Here's how the part is built. I have some questions about the finished solid (model axes, mm). Face numbers are marked on the shaded views. A direction names the side the tool comes from. Round coordinates to 2 decimals unless told otherwise and drop trailing zeros. Order: outer loops, then holes, each group sorted by start corner. A loop starts at its lowest first (then second) coordinate and runs counter-clockwise, first axis right, second up. Notation, with made-up numbers: (47, 11) - (105, 11) arc R26 ccw to (105, 42) - close; hole circle Ø10 at (42, 5.5). An arc over 180 degrees is marked (long way). One line per item, written item: value.
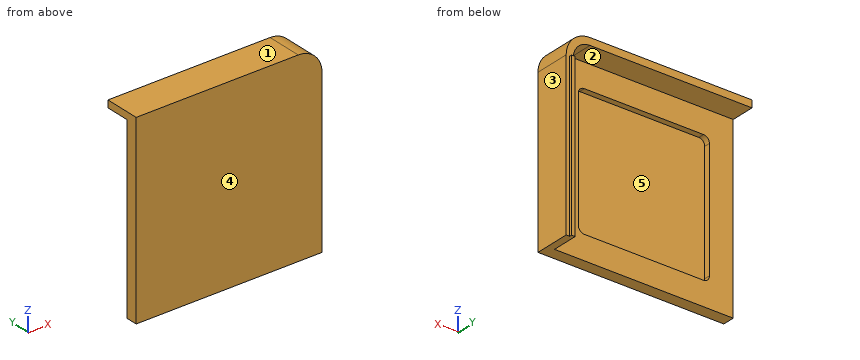
from build123d import *

# Parameters (mm, degrees)
SKIZZE9_W               = 156
SKIZZE9_H               = 156
SKIZZE9_W_2             = 110
SKIZZE9_H_2             = 110
LINEAR_AUSTRAGEN4_DEPTH = 5
VERRUNDUNG5_R           = 5
SKIZZE10_W              = 156
SKIZZE10_H              = 156
LINEAR_AUSTRAGEN5_DEPTH = 5
LINEAR_AUSTRAGEN6_DEPTH = 20
VERRUNDUNG6_R           = 20
VERRUNDUNG7_R           = 14
SKIZZE12_W              = 3
SKIZZE12_H              = 136
LINEAR_AUSTRAGEN7_DEPTH = 2


with BuildPart() as part:
    # Skizze9 → Linear austragen4 (new body)
    with BuildSketch(Plane(origin=(0, 0, 0), x_dir=(1, 0, 0), z_dir=(0, 1, 0))):
        with Locations((78, 78)):
            Rectangle(SKIZZE9_W, SKIZZE9_H)
        with Locations((75, 81)):
            Rectangle(SKIZZE9_W_2, SKIZZE9_H_2, mode=Mode.SUBTRACT)
    extrude(amount=LINEAR_AUSTRAGEN4_DEPTH)

    # Verrundung5
    verrundung5_edges = [part.edges().sort_by_distance(p)[0] for p in [
        (20, 2.5, -136),
        (20, 2.5, -26),
        (130, 2.5, -26),
        (130, 2.5, -136),
    ]]
    fillet(verrundung5_edges, radius=VERRUNDUNG5_R)

    # Skizze10 → Linear austragen5 (add)
    with BuildSketch(Plane.XZ):
        with Locations((78, -78)):
            Rectangle(SKIZZE10_W, SKIZZE10_H)
    extrude(amount=LINEAR_AUSTRAGEN5_DEPTH)

    # Skizze11 → Linear austragen6 (add)
    with BuildSketch(Plane(origin=(0, 5, 0), x_dir=(1, 0, 0), z_dir=(0, 1, 0))):
        Polygon((0, 0), (156, 0), (156, 156), (150, 156), (150, 6), (0, 6), align=None)
    extrude(amount=LINEAR_AUSTRAGEN6_DEPTH)

    # Verrundung6
    verrundung6_edges = [part.edges().sort_by_distance(p)[0] for p in [
        (156, 10, 0),
    ]]
    fillet(verrundung6_edges, radius=VERRUNDUNG6_R)

    # Verrundung7
    verrundung7_edges = [part.edges().sort_by_distance(p)[0] for p in [
        (150, 15, -6),
    ]]
    fillet(verrundung7_edges, radius=VERRUNDUNG7_R)

    # Skizze12 → Linear austragen7 (add)
    with BuildSketch(Plane(origin=(0, 25, 0), x_dir=(1, 0, 0), z_dir=(0, 1, 0))):
        with Locations((151.5, 88)):
            Rectangle(SKIZZE12_W, SKIZZE12_H)
    extrude(amount=LINEAR_AUSTRAGEN7_DEPTH)


solid = part.part
Q1. If we section it at A-A, the plane z = -111: Please give me the cut outline in (x, y).
Results list:
outline: (0, -5) - (156, -5) - (156, 25) - (153, 25) - (153, 27) - (150, 27) - (150, 5) - (130, 5) - (130, 0) - (20, 0) - (20, 5) - (0, 5) - close
Q2. We'd pull the mould along X, two halves only. Please class the marked faces 3, 4 and 5: released by +X, released by -X, zero draft, split by the parting line, or undercut.
Results list:
face 3: released by +X
face 4: zero draft
face 5: undercut
Q3. If we section it at D-D, the plane x = 132: Please give me the cut outline in (y, z), then the cut area to 3 significant figures.
Results list:
outline: (-5, -156) - (5, -156) - (5, -6) - (25, -6) - (25, 0) - (-5, 0) - close
area: 1,680 mm²
Q4. Will these pins go through, and if not, where does the flat tip stop? pin 1 (2 mm diameter, centred on x = 151.5, y = 25.5, fed in from +Z); pin 2 (12 mm diameter, centred on x = 40, z = -74, fed in from +Y); pin 3 (6 mm diameter, centred on y = 10.5, z = -136, fed in from -X).
Results list:
pin 1: z = -6.37
pin 2: y = 0
pin 3: x = 150
Q5. If I drill on line 1 along Y through (x, z) = (26.5, -113); line 2 along Y through (x, z) = (139, -114.5); line 3 along X through (y, z) = (1.5, -37), over which ranges is the centre line in solid material (lowest first)?
Results list:
line 1: -5 to 0
line 2: -5 to 5
line 3: 0 to 20, 130 to 156
Q6. Which directions (+Z, -Z, +X, -X, +Y, -Y) give clear straight access to the entire face, cutting with the end or side of a thin tool? Please do the marked faces 1 and 2.
Results list:
face 1: +Z, +X, -X, +Y, -Y
face 2: -Z, -X, +Y
Q7. If we section it at C-C, the plane y = 7: Please give me the cut outline in (x, z), then the cut area to 3 significant figures.
Results list:
outline: (0, -6) - (136, -6) arc R14 cw to (150, -20) - (150, -156) - (156, -156) - (156, -20) arc R20 ccw to (136, 0) - (0, 0) - close
area: 1,790 mm²
Q8. If we section it at B-B, the plane x = 112: Please give me the cut outline in (y, z).
Results list:
outline: (-5, -156) - (5, -156) - (5, -136) - (0, -136) - (0, -26) - (5, -26) - (5, -6) - (25, -6) - (25, 0) - (-5, 0) - close
